Work out the finished part from the listing and answer in its coordinate system (mm). Coordinates: 2 decimals unless noted, no trailing zeros. Write each loop counter-clockwise with the first axis right and the second up, starting at its lowest first coordinate (ties: lowest second). Pieces come first, ordered by that corner, then holes. Notation, with made-up numbers: (76.25, -36) - (131.25, -36) arc R7 ccw to (131.25, -30) - close; hole circle Ø4 at (3.5, -22.75). An arc over 180 degrees is marked (long way). Use one line per item in the form item = value. Start each with the question number.
Item 1: A cutting plane is placed at B-B (x = -139.5). Write down the section's boundary in (y, z).
Item 2: A cutting plane is placed at A-A (y = 73). Write down the section's boundary in (x, z), then the cut area to 3 significant figures.
Item 3: Given pin 1 (12 mm diameter, centred on x = 45.5, z = -23, fed in from +Y); pin 2 (5 mm diameter, centred on x = 137.5, y = 134, fed in from +Z), each flat-ended and moving along its own axis, determine where each tip first touches the part or whether it passes through.
Item 4: A cutting plane is placed at D-D (z = 25). Write down the section's boundary in (x, y).
Item 5: A cutting plane is placed at C-C (z = 139.5). Write down the section's boundary in (x, y), then the cut area to 3 significant figures.
Item 6: Consider probe 1 along X at (y, z) = (115, -138.5); probe 2 along Y at (x, z) = (-221.5, -36.5). Determine where each line is inside the solid, lowest interval first.
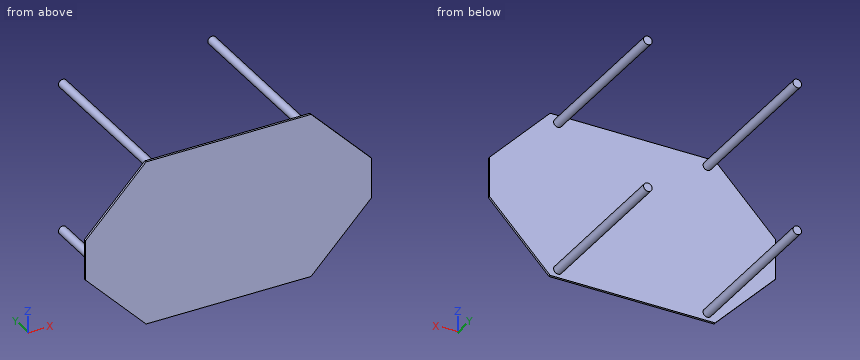
from build123d import *

# Parameters (mm, degrees)
EXTRUDE_2_DEPTH = 4
SKETCH_2_R      = 8
EXTRUDE_3_DEPTH = 300


with BuildPart() as part:
    # Эскиз1 → Бобышка-Вытянуть2 (new body)
    with BuildSketch(Plane(origin=(0, 0, 0), x_dir=(1, 0, 0), z_dir=(0, 1, 0))):
        Polygon((154, -154), (-154, -154), (-267, -37.5), (-267, 37.5), (-154, 154), (154, 154), (267, 37.5), (267, -37.5), align=None)
    extrude(amount=-EXTRUDE_2_DEPTH)

    # Эскиз2 → Бобышка-Вытянуть3 (add)
    with BuildSketch(Plane(origin=(0, 0, 0), x_dir=(1, 0, 0), z_dir=(0, 1, 0))):
        with Locations(Location((-139.5, 139.5, 0), (0, 0, 270))):
            Circle(SKETCH_2_R)
        with Locations(Location((139.5, 139.5, 0), (0, 0, 90))):
            Circle(SKETCH_2_R)
        with Locations(Location((139.5, -139.5, 0), (0, 0, 270))):
            Circle(SKETCH_2_R)
        with Locations(Location((-139.5, -139.5, 0), (0, 0, 90))):
            Circle(SKETCH_2_R)
    extrude(amount=EXTRUDE_3_DEPTH)


solid = part.part
Answer:
q1.outline = (-4, -154) - (0, -154) - (0, -147.5) - (300, -147.5) - (300, -131.5) - (0, -131.5) - (0, 131.5) - (300, 131.5) - (300, 147.5) - (0, 147.5) - (0, 154) - (-4, 154) - close
q2.outline = circle Ø16 at (-139.5, -139.5); circle Ø16 at (-139.5, 139.5); circle Ø16 at (139.5, -139.5); circle Ø16 at (139.5, 139.5)
q2.area = 804 mm²
q3.pin_1 = 0
q3.pin_2 = 147.5
q4.outline = (-267, -4) - (267, -4) - (267, 0) - (-267, 0) - close
q5.outline = (-168.06, -4) - (168.06, -4) - (168.06, 0) - (147.5, 0) - (147.5, 300) - (131.5, 300) - (131.5, 0) - (-131.5, 0) - (-131.5, 300) - (-147.5, 300) - (-147.5, 0) - (-168.06, 0) - close
q5.area = 10,900 mm²
q6.probe_1 = -147.44 to -131.56, 131.56 to 147.44
q6.probe_2 = -4 to 0
